Job drawing, mm, ordinate dimensions from the low corner. One solid piece. A direction names the side the tool comes from. Coordinates: 2 decimals unless noted, no trailing zeros. Loops run counter-clockwise (first coordinate to the right, second up) from the corner with the lowest first, then second, coordinate; pieces in that order, holes last. Notation, with made-up numbers: (88, 22.25) - (139, 22.25) arc R25 ccw to (139, 36.25) - close; hole circle Ø5 at (75.25, 14). An arc over 180 degrees is marked (long way). Use a Markdown table: item, result. Add a question column.
1) Band-saw the part on D-D (y = 5.75). Give the cut face in (x, z) (1 decimal).
2) Band-saw the part on C-C (x = 8). Give the cut face in (y, z) (1 decimal), plus the area to 3 significant figures.
3) Band-saw the part on B-B (z = 24.5). Give the cut face in (x, y), plus the area to 3 significant figures.
4) Tool access for the marked faces 4, 5, 6 and 7: list every direction of +Z, -Z, +X, -X, +Y, -Y with a clear straight run to the whole face (end or side of a thin tool).
5) Band-saw the part on A-A (x = 24.5). Give the cut face in (y, z).
6) Probe probe 1 along Y at (x, z) = (24.5, 8.15); probe 2 along Z at (x, y) = (30, 2). List the from-to ranges inside material, lowest first. Write a range as [from, to].
7) Pull direction X, two halves, no side cores. Call the marked faces 1, 2 and 3: +X half, -X half, draft (parallel to the pull), parting line (faces both ways), or undercut.
8) Drop flat-ended pins along their axis: P1, Ø4, axis at x = 20, y = 8.5, coming from the -Z side; P2, Ø5, axis at y = 6, z = 24.5, coming from the +X side; P3, Ø5, axis at x = 4, z = 17, coming from the -Y side; P4, Ø1, axis at x = 6, y = 6.5, coming from the +Z side. Give the stop position or say it passes through.
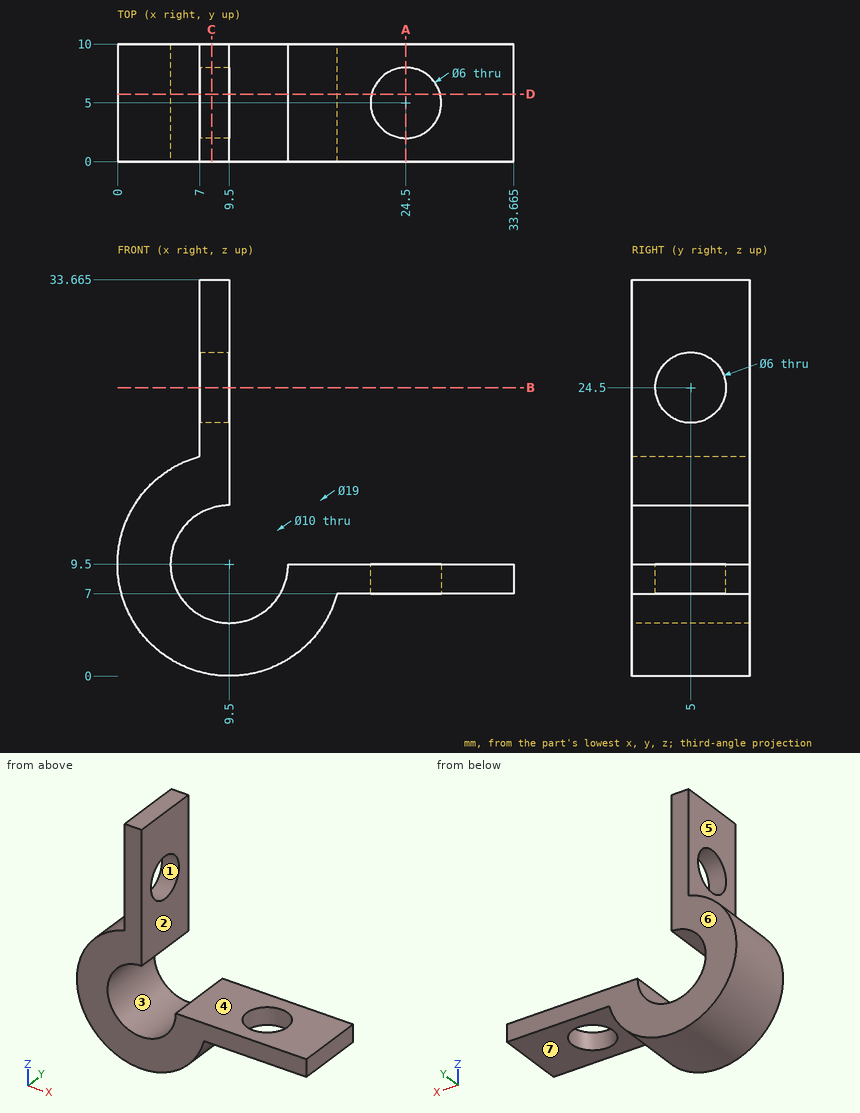
Answer block:
| question | item | result |
|---|---|---|
| 1 | outline | (7, 18.7) arc R9.5 ccw (long way) to (18.7, 7) - (21.6, 7) - (21.6, 9.5) - (14.5, 9.5) arc R5 cw (long way) to (9.5, 14.5) - (9.5, 21.6) - (7, 21.6) - close; (7, 27.4) - (9.5, 27.4) - (9.5, 33.7) - (7, 33.7) - close; (27.4, 7) - (33.7, 7) - (33.7, 9.5) - (27.4, 9.5) - close |
| 2 | outline | (0, 0.1) - (10, 0.1) - (10, 4.7) - (0, 4.7) - close; (0, 14.3) - (10, 14.3) - (10, 33.7) - (0, 33.7) - close; hole circle Ø6 at (5, 24.5) |
| 2 | area | 212 mm2 |
| 3 | outline | (7, 0) - (9.5, 0) - (9.5, 2) - (7, 2) - close; (7, 8) - (9.5, 8) - (9.5, 10) - (7, 10) - close |
| 3 | area | 10.0 mm2 |
| 4 | face 4 | +Z, +X, +Y, -Y |
| 4 | face 5 | +Z, -X, +Y, -Y |
| 4 | face 6 | +Z, -Z, +X, -X, +Y |
| 4 | face 7 | -Z, +X, +Y, -Y |
| 5 | outline | (0, 7) - (2, 7) - (2, 9.5) - (0, 9.5) - close; (8, 7) - (10, 7) - (10, 9.5) - (8, 9.5) - close |
| 6 | probe 1 | [0, 2], [8, 10] |
| 6 | probe 2 | [7, 9.5] |
| 7 | face 1 | draft |
| 7 | face 2 | +X half |
| 7 | face 3 | undercut |
| 8 | P1 | z = 5.26 |
| 8 | P2 | x = 9.5 |
| 8 | P3 | y = 0 |
| 8 | P4 | z = 18.51 |
